from build123d import *

# Parameters (mm, degrees)
SKETCH_1_W      = 9
SKETCH_1_H      = 9
EXTRUDE_1_DEPTH = 27
SKETCH_2_R      = 4
EXTRUDE_2_DEPTH = 7
SKETCH_3_R      = 5.25
EXTRUDE_3_DEPTH = 37


with BuildPart() as part:
    # 草图1 → 凸台-拉伸1 (new body)
    with BuildSketch(Plane.XY):
        with Locations((-4.5, 4.5)):
            Rectangle(SKETCH_1_W, SKETCH_1_H)
    extrude(amount=EXTRUDE_1_DEPTH)

    # 草图2 → 凸台-拉伸2 (add)
    with BuildSketch(Plane.XZ):
        with Locations((-4.5, 3.5)):
            Circle(SKETCH_2_R)
    extrude(amount=EXTRUDE_2_DEPTH)

    # 草图3 → 凸台-拉伸3 (add)
    with BuildSketch(Plane.XZ.offset(7)):
        with Locations((-4.5, 3.5)):
            Circle(SKETCH_3_R)
    extrude(amount=EXTRUDE_3_DEPTH)


solid = part.part
Work out the finished part from the listing and answer in its coordinate system (mm). A direction names the side the tool comes from. Give positions to 0.01 mm unless a question says otherwise; leave off trailing zeros. Order: outer loops, then holes, each group sorted by start corner. A loop starts at its lowest first (then second) coordinate and runs counter-clockwise, first axis right, second up. Notation, with made-up numbers: (39.25, 85) -> (52.25, 85) arc R26 ccw to (52.25, 100) -> close; hole circle Ø8 at (14.5, -17). An arc over 180 degrees is marked (long way). One line per item, written item: value.
Item 1: Flat-ended cylindrical pins translate along their axes: P1, Ø6, axis at x = -4.5, z = 13.5, coming from the -Y side; P2, Ø10, axis at y = 5.5, z = 7, coming from the +X side; P3, Ø1, axis at x = -2, y = -8, coming from the +Z side. Find the tip coordinate at first contact, or state that the pin passes through.
Answer sheet:
P1: y = 0
P2: x = 0
P3: z = 8.35
Item 2: Determine the mould class of faces 4 (the flat face through (-5, 5, 27)), 5 (the cylindrical face through (-5.367, -3.451, -0.405)), 6 (the flat face through (-5, -44, 4)) for opening direction Y: released by +Y, released by -Y, zero draft, split by the parting line, or undercut.
Answer sheet:
face 4: zero draft
face 5: undercut
face 6: released by -Y
Item 3: Straight lines are drawn through the part: probe 1 along X at (y, z) = (6.5, 20.75); probe 2 along Z at (x, y) = (-4.5, -38.5); probe 3 along Y at (x, z) = (-1, 17.75). For each, find the intervals that lie inside material, in ascending order.
Answer sheet:
probe 1: -9 to 0
probe 2: -1.75 to 8.75
probe 3: 0 to 9
Item 4: Find section A-A, the plane x = -4.5. Give the vertices of the cut face in (y, z).
Answer sheet:
outline: (-44, -1.75) -> (-7, -1.75) -> (-7, -0.5) -> (0, -0.5) -> (0, 0) -> (9, 0) -> (9, 27) -> (0, 27) -> (0, 7.5) -> (-7, 7.5) -> (-7, 8.75) -> (-44, 8.75) -> close
Item 5: Find section C-C, the plane y = -29.5. Give the vertices of the cut face in (x, z).
Answer sheet:
outline: circle Ø10.5 at (-4.5, 3.5)
Item 6: Find section B-B, the plane z = 3.5. Give the vertices of the cut face in (x, y), plus the area to 4 significant figures.
Answer sheet:
outline: (-9.75, -44) -> (0.75, -44) -> (0.75, -7) -> (-0.5, -7) -> (-0.5, 0) -> (0, 0) -> (0, 9) -> (-9, 9) -> (-9, 0) -> (-8.5, 0) -> (-8.5, -7) -> (-9.75, -7) -> close
area: 525.5 mm²
Item 7: A tool of negligible diameter and unlimited length cuts with its end or side. For faces 1 (the flat face through (-3, -7, -0.4)), 2 (the flat face through (-9, 4, 13)), 3 (the flat face through (-5, 5, 0)), from which of +Z, -Z, +X, -X, +Y, -Y can it reach the whole face along a straight path? Write none if from no direction.
Answer sheet:
face 1: none
face 2: +Z, -Z, -X, +Y
face 3: -Z, +X, -X, +Y
Item 8: Find section D-D, the plane z = 16.75. Give the vertices of the cut face in (x, y), plus the area to 3 significant figures.
Answer sheet:
outline: (-9, 0) -> (0, 0) -> (0, 9) -> (-9, 9) -> close
area: 81.0 mm²
